The listing builds one solid part. Answer for the finished solid, in the listing's coordinates (mm). A direction names the side the tool comes from. Coordinates: 2 decimals unless noted, no trailing zeros. Loops run counter-clockwise (first coordinate to the right, second up) from the corner with the lowest first, then second, coordinate; pieces in that order, holes last. Notation, with made-up numbers: (59, -1) - (84, -1) arc R19 ccw to (84, 6) - close; hole circle Ø3 at (56, 74). An arc over 180 degrees is marked (long way). One line per question, with ' | ' between items.
from build123d import *

# Parameters (mm, degrees)
GRUNDK_RPER_DEPTH = 1.8
L_FTUNGEN_DEPTH   = 1.8
SKIZZE4_W         = 2
SKIZZE4_H         = 69.501766887
STREBE_DEPTH      = 1


with BuildPart() as part:
    # Skizze2 → Grundkörper (new body)
    with BuildSketch(Plane(origin=(0, 0, 0), x_dir=(1, 0, 0), z_dir=(0, 1, 0))):
        with BuildLine():
            Line((-43.5, 50), (-27.5, 50))
            Line((-27.5, 50), (-17.028881642, 33))
            ThreePointArc((-17.028881642, 33), (0, 23.488907952), (17.028881642, 33))
            Line((17.028881642, 33), (27.5, 50))
            Line((27.5, 50), (43.5, 50))
            ThreePointArc((43.5, 50), (47.035533906, 48.535533906), (48.5, 45))
            Line((48.5, 45), (48.5, -49))
            Line((48.5, -49), (-48.5, -49))
            Line((-48.5, -49), (-48.5, 45))
            ThreePointArc((-48.5, 45), (-47.035533906, 48.535533906), (-43.5, 50))
        make_face()
    extrude(amount=GRUNDK_RPER_DEPTH)

    # Skizze3 → Lüftungen (cut)
    with BuildSketch(Plane(origin=(0, 1.8, 0), x_dir=(1, 0, 0), z_dir=(0, 1, 0))):
        with BuildLine():
            Line((-39.25, 15), (-5.75, 15))
            ThreePointArc((-5.75, 15), (-4.335786438, 14.414213562), (-3.75, 13))
            Line((-3.75, 13), (-3.75, 9))
            ThreePointArc((-3.75, 9), (-4.335786438, 7.585786438), (-5.75, 7))
            Line((-5.75, 7), (-39.25, 7))
            ThreePointArc((-39.25, 7), (-40.664213562, 7.585786438), (-41.25, 9))
            Line((-41.25, 9), (-41.25, 13))
            ThreePointArc((-41.25, 13), (-40.664213562, 14.414213562), (-39.25, 15))
        make_face()
        with BuildLine():
            Line((3.75, 13), (3.75, 9))
            ThreePointArc((3.75, 9), (4.335786438, 7.585786438), (5.75, 7))
            Line((5.75, 7), (39.25, 7))
            ThreePointArc((39.25, 7), (40.664213562, 7.585786438), (41.25, 9))
            Line((41.25, 9), (41.25, 13))
            ThreePointArc((41.25, 13), (40.664213562, 14.414213562), (39.25, 15))
            Line((39.25, 15), (5.75, 15))
            ThreePointArc((5.75, 15), (4.335786438, 14.414213562), (3.75, 13))
        make_face()
        with BuildLine():
            Line((3.75, 1), (3.75, -3))
            ThreePointArc((3.75, -3), (4.335786438, -4.414213562), (5.75, -5))
            Line((5.75, -5), (39.25, -5))
            ThreePointArc((39.25, -5), (40.664213562, -4.414213562), (41.25, -3))
            Line((41.25, -3), (41.25, 1))
            ThreePointArc((41.25, 1), (40.664213562, 2.414213562), (39.25, 3))
            Line((39.25, 3), (5.75, 3))
            ThreePointArc((5.75, 3), (4.335786438, 2.414213562), (3.75, 1))
        make_face()
        with BuildLine():
            Line((3.75, -11), (3.75, -15))
            ThreePointArc((3.75, -15), (4.335786438, -16.414213562), (5.75, -17))
            Line((5.75, -17), (39.25, -17))
            ThreePointArc((39.25, -17), (40.664213562, -16.414213562), (41.25, -15))
            Line((41.25, -15), (41.25, -11))
            ThreePointArc((41.25, -11), (40.664213562, -9.585786438), (39.25, -9))
            Line((39.25, -9), (5.75, -9))
            ThreePointArc((5.75, -9), (4.335786438, -9.585786438), (3.75, -11))
        make_face()
        with BuildLine():
            Line((3.75, -23), (3.75, -27))
            ThreePointArc((3.75, -27), (4.335786438, -28.414213562), (5.75, -29))
            Line((5.75, -29), (39.25, -29))
            ThreePointArc((39.25, -29), (40.664213562, -28.414213562), (41.25, -27))
            Line((41.25, -27), (41.25, -23))
            ThreePointArc((41.25, -23), (40.664213562, -21.585786438), (39.25, -21))
            Line((39.25, -21), (5.75, -21))
            ThreePointArc((5.75, -21), (4.335786438, -21.585786438), (3.75, -23))
        make_face()
        with BuildLine():
            Line((3.75, -35), (3.75, -39))
            ThreePointArc((3.75, -39), (4.335786438, -40.414213562), (5.75, -41))
            Line((5.75, -41), (39.25, -41))
            ThreePointArc((39.25, -41), (40.664213562, -40.414213562), (41.25, -39))
            Line((41.25, -39), (41.25, -35))
            ThreePointArc((41.25, -35), (40.664213562, -33.585786438), (39.25, -33))
            Line((39.25, -33), (5.75, -33))
            ThreePointArc((5.75, -33), (4.335786438, -33.585786438), (3.75, -35))
        make_face()
        with BuildLine():
            Line((-41.25, 1), (-41.25, -3))
            ThreePointArc((-41.25, -3), (-40.664213562, -4.414213562), (-39.25, -5))
            Line((-39.25, -5), (-5.75, -5))
            ThreePointArc((-5.75, -5), (-4.335786438, -4.414213562), (-3.75, -3))
            Line((-3.75, -3), (-3.75, 1))
            ThreePointArc((-3.75, 1), (-4.335786438, 2.414213562), (-5.75, 3))
            Line((-5.75, 3), (-39.25, 3))
            ThreePointArc((-39.25, 3), (-40.664213562, 2.414213562), (-41.25, 1))
        make_face()
        with BuildLine():
            Line((-41.25, -11), (-41.25, -15))
            ThreePointArc((-41.25, -15), (-40.664213562, -16.414213562), (-39.25, -17))
            Line((-39.25, -17), (-5.75, -17))
            ThreePointArc((-5.75, -17), (-4.335786438, -16.414213562), (-3.75, -15))
            Line((-3.75, -15), (-3.75, -11))
            ThreePointArc((-3.75, -11), (-4.335786438, -9.585786438), (-5.75, -9))
            Line((-5.75, -9), (-39.25, -9))
            ThreePointArc((-39.25, -9), (-40.664213562, -9.585786438), (-41.25, -11))
        make_face()
        with BuildLine():
            Line((-41.25, -23), (-41.25, -27))
            ThreePointArc((-41.25, -27), (-40.664213562, -28.414213562), (-39.25, -29))
            Line((-39.25, -29), (-5.75, -29))
            ThreePointArc((-5.75, -29), (-4.335786438, -28.414213562), (-3.75, -27))
            Line((-3.75, -27), (-3.75, -23))
            ThreePointArc((-3.75, -23), (-4.335786438, -21.585786438), (-5.75, -21))
            Line((-5.75, -21), (-39.25, -21))
            ThreePointArc((-39.25, -21), (-40.664213562, -21.585786438), (-41.25, -23))
        make_face()
        with BuildLine():
            Line((-41.25, -35), (-41.25, -39))
            ThreePointArc((-41.25, -39), (-40.664213562, -40.414213562), (-39.25, -41))
            Line((-39.25, -41), (-5.75, -41))
            ThreePointArc((-5.75, -41), (-4.335786438, -40.414213562), (-3.75, -39))
            Line((-3.75, -39), (-3.75, -35))
            ThreePointArc((-3.75, -35), (-4.335786438, -33.585786438), (-5.75, -33))
            Line((-5.75, -33), (-39.25, -33))
            ThreePointArc((-39.25, -33), (-40.664213562, -33.585786438), (-41.25, -35))
        make_face()
    extrude(amount=-L_FTUNGEN_DEPTH, mode=Mode.SUBTRACT)

    # Skizze4 → Strebe (add)
    with BuildSketch(Plane(origin=(0, 1.8, 0), x_dir=(1, 0, 0), z_dir=(0, 1, 0))):
        with Locations((0, -12.068236179)):
            Rectangle(SKIZZE4_W, SKIZZE4_H)
    extrude(amount=STREBE_DEPTH)


solid = part.part
Item 1: Find section C-C, the plane y = 0.7. State how many separate pieces and enclosed holes the cut face has, plus the area to 3 significant figures.
Taken from the geometry:
separate pieces: 1 | enclosed holes: 10 | area: 5,640 mm2
Item 2: Which of the six approach directions +Z, -Z, +X, -X, +Y, -Y give full straight-line access (tool end or side, diameter ignored) to faces 1 (the face through (1, 0, 10)), 2 (the face through (22.19, 0.89, -41.38))?
Taken from the geometry:
face 1: +Z, -Z, +X, -X, -Y | face 2: -Z, +Y, -Y
Item 3: Find section A-A, the plane z = 37.5. Write down the section's boundary in (x, y), plus the area to 3 significant figures.
Taken from the geometry:
outline: (-48.5, 0) - (-41.25, 0) - (-41.25, 1.8) - (-48.5, 1.8) - close; (-3.75, 0) - (3.75, 0) - (3.75, 1.8) - (1, 1.8) - (1, 2.8) - (-1, 2.8) - (-1, 1.8) - (-3.75, 1.8) - close; (41.25, 0) - (48.5, 0) - (48.5, 1.8) - (41.25, 1.8) - close | area: 41.6 mm2
Item 4: Find the intervals of material crossed by line 1 (X direction, y = 0.2, z = 1.5); line 2 (Z direction, x = 34.5, y = 0.25); line 3 (Z direction, x = 18.5, y = 0.6), in increasing order. Write a range as [from, to].
Taken from the geometry:
line 1: x = [-48.5, -41.25], [-3.75, 3.75], [41.25, 48.5] | line 2: z = [-50, -15], [-7, -3], [5, 9], [17, 21], [29, 33], [41, 49] | line 3: z = [-35.39, -15], [-7, -3], [5, 9], [17, 21], [29, 33], [41, 49]
Item 5: The mould has two halves that part along X. Classify faces 3 (the face through (-0.29, 0.89, -23.49)), 4 (the face through (47, 0.89, -48.57)), 5 (the face through (-47.07, 0.89, -48.5)): pulls with the +X half, pulls with the -X half, needs draft (parallel to the pull), parting line crosses it, or undercut.
Taken from the geometry:
face 3: undercut | face 4: pulls with the +X half | face 5: pulls with the -X half
Item 6: Find section B-B, the plane x = 38. Write down the section's boundary in (y, z), plus the area to 3 significant figures.
Taken from the geometry:
outline: (0, -50) - (1.8, -50) - (1.8, -15) - (0, -15) - close; (0, -7) - (1.8, -7) - (1.8, -3) - (0, -3) - close; (0, 5) - (1.8, 5) - (1.8, 9) - (0, 9) - close; (0, 17) - (1.8, 17) - (1.8, 21) - (0, 21) - close; (0, 29) - (1.8, 29) - (1.8, 33) - (0, 33) - close; (0, 41) - (1.8, 41) - (1.8, 49) - (0, 49) - close | area: 106 mm2
Item 7: Each of these flat-tipped pins is pushed along its axis until it touches: pin 1 Ø0.5 at (x, y) = (27, 0.5) entering from -Z; pin 2 Ø4 at (x, z) = (34, 30.5) entering from +Y; pin 3 Ø0.5 at (y, z) = (2.5, 27.5) entering from +X. Where does it stop, or does it pass through?
Taken from the geometry:
pin 1: stops at z = -49.59 | pin 2: stops at y = 1.8 | pin 3: stops at x = 1
Item 8: Find section D-D, the plane x = -20.5. Write down the section's boundary in (y, z), plus the area to 3 significant figures.
Taken from the geometry:
outline: (0, -38.64) - (1.8, -38.64) - (1.8, -15) - (0, -15) - close; (0, -7) - (1.8, -7) - (1.8, -3) - (0, -3) - close; (0, 5) - (1.8, 5) - (1.8, 9) - (0, 9) - close; (0, 17) - (1.8, 17) - (1.8, 21) - (0, 21) - close; (0, 29) - (1.8, 29) - (1.8, 33) - (0, 33) - close; (0, 41) - (1.8, 41) - (1.8, 49) - (0, 49) - close | area: 85.7 mm2
